```python
from build123d import *

# Parameters (mm, degrees)
F0_W     = 36
F0_H     = 30.441777
F1_DEPTH = 23
F3_DEPTH = 25
F5_DEPTH = 91


with BuildPart() as f1:
    # F0 (on Top) → F1 (new body)
    with BuildSketch(Plane.XY):
        with Locations((0, 15.220888)):
            Rectangle(F0_W, F0_H)
        Polygon((18, 0), (-18, 0), (-33, 0), (-33, -40), (33, -40), (33, 0), align=None)
    extrude(amount=F1_DEPTH)

    # F2 (on face) → F3 (join)
    with BuildSketch(Plane.YZ.offset(33)):
        Polygon((-27.114989, 13), (-28.644967, 13), (-29.409956, 11.675), (-28.644967, 10.35), (-27.114989, 10.35), (-26.35, 11.675), align=None)
    extrude(amount=F3_DEPTH)

    # F4 (on face) → F5 (join)
    with BuildSketch(Plane.YZ.offset(33)):
        Polygon((-27.114989, 13), (-28.644967, 13), (-29.409956, 11.675), (-28.644967, 10.35), (-27.114989, 10.35), (-26.35, 11.675), align=None)
    extrude(amount=-F5_DEPTH)


solid = f1.part
```
The model under review builds one solid part; all positions refer to its coordinate system, in mm. A direction names the side the tool comes from. Give positions to 0.01 mm unless a question says otherwise; leave off trailing zeros. Loops run counter-clockwise (first coordinate to the right, second up) from the corner with the lowest first, then second, coordinate; pieces in that order, holes last. Notation, with made-up numbers: (52, 16.5) -> (78, 16.5) arc R15 cw to (78, 31.5) -> close; hole circle Ø11 at (51, 61). An arc over 180 degrees is marked (long way). Use CSV: the item, a comma, the result in double quotes.
1. Consider section C-C, the plane y = 8.5. Write out the cut boundary in (x, z).
Result:
outline,"(-18, 0) -> (18, 0) -> (18, 23) -> (-18, 23) -> close"
2. Consider section D-D, the plane y = -11.5. Write out the cut boundary in (x, z).
Result:
outline,"(-33, 0) -> (33, 0) -> (33, 23) -> (-33, 23) -> close"
3. To check wall thickness, follow probe 1 along Y at (x, z) = (20.5, 17.5); probe 2 along X at (y, z) = (-24.5, 7.75); probe 3 along X at (y, z) = (8.5, 7.25). State the ranges of each line that lie inside material, in increasing order. Write a range as from..to.
Result:
probe 1,"y = -40..0"
probe 2,"x = -33..33"
probe 3,"x = -18..18"
4. Consider section A-A, the plane z = 15.75. Write out the cut boundary in (x, y).
Result:
outline,"(-33, -40) -> (33, -40) -> (33, 0) -> (18, 0) -> (18, 30.44) -> (-18, 30.44) -> (-18, 0) -> (-33, 0) -> close"
5. For P1, Ø1.7, axis at x = -50.5, y = -27.5, coming from the -Z side; P2, Ø4, axis at y = 5, z = 7, coming from the -X side; P3, Ø1.2, axis at x = 45.5, y = -27.5, coming from the +Z side, all flat-tipped, find the tip position at first contact; note any pin that passes through.
Result:
P1,"stops at z = 10.35"
P2,"stops at x = -18"
P3,"stops at z = 13"
6. Machinability: for faces 1 (the face through (26, 0, 11)), 2 (the face through (0, 30.442, 11)), 3 (the face through (-25, 0, 11)), which of the approach directions +Z, -Z, +X, -X, +Y, -Y give a long, thin tool a straight path to every point of the face, cutting with its end or side? Answer none if there is none.
Result:
face 1,"+Z, -Z, +X, +Y"
face 2,"+Z, -Z, +X, -X, +Y"
face 3,"+Z, -Z, -X, +Y"
7. Consider section B-B, the plane x = 39.5. Write out the cut boundary in (y, z) (3 decimals), then the cut area to 3 significant figures.
Result:
outline,"(-29.41, 11.675) -> (-28.645, 10.35) -> (-27.115, 10.35) -> (-26.35, 11.675) -> (-27.115, 13) -> (-28.645, 13) -> close"
area,"6.08 mm²"
